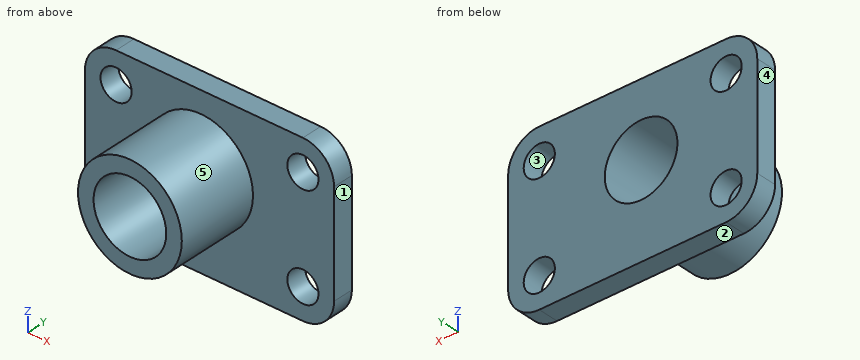
from build123d import *

# Parameters (mm, degrees)
F0_R     = 25
F0_R_2   = 17.5
F1_DEPTH = 50
F2_DEPTH = 112
F0_R_3   = 7.5
F3_DEPTH = 10


# Not quite as in the source:
# - an extrude ends at something that could not be found from the text; its depth is read off the source's solid


with BuildPart() as f1:
    # F0 (on Front) → F1 (new body)
    with BuildSketch(Plane.XZ):
        Circle(F0_R)
        Circle(F0_R_2, mode=Mode.SUBTRACT)
    extrude(amount=F1_DEPTH)

    # F0 (on Front) → F2 (cut, through all)
    with BuildSketch(Plane.XZ):
        Circle(F0_R_2)
    extrude(amount=-F2_DEPTH, mode=Mode.SUBTRACT)

    # F0 (on Front) → F3 (join)
    with BuildSketch(Plane.XZ):
        with BuildLine():
            Line((49.0495060384, 35.4441977432), (-40.9504939616, 35.4441977432))
            ThreePointArc((-40.9504939616, 35.4441977432), (-51.5570956794, 31.050799461), (-55.9504939616, 20.4441977432))
            Line((-55.9504939616, 20.4441977432), (-55.9504939616, -29.5558022568))
            ThreePointArc((-55.9504939616, -29.5558022568), (-51.5570956794, -40.1624039746), (-40.9504939616, -44.5558022568))
            Line((-40.9504939616, -44.5558022568), (49.0495060384, -44.5558022568))
            ThreePointArc((49.0495060384, -44.5558022568), (59.6561077562, -40.1624039746), (64.0495060384, -29.5558022568))
            Line((64.0495060384, -29.5558022568), (64.0495060384, 20.4441977432))
            ThreePointArc((64.0495060384, 20.4441977432), (59.6561077562, 31.050799461), (49.0495060384, 35.4441977432))
        make_face()
        with Locations((-40.9504939616, -29.5558022568)):
            Circle(F0_R_3, mode=Mode.SUBTRACT)
        with Locations((49.0495060384, -29.5558022568)):
            Circle(F0_R_3, mode=Mode.SUBTRACT)
        Circle(F0_R, mode=Mode.SUBTRACT)
        with Locations((-40.9504939616, 20.4441977432)):
            Circle(F0_R_3, mode=Mode.SUBTRACT)
        with Locations((49.0495060384, 20.4441977432)):
            Circle(F0_R_3, mode=Mode.SUBTRACT)
    extrude(amount=F3_DEPTH)


solid = f1.part
Verification items for the finished model (mm, model axes). Face numbers are marked on the shaded views. A direction names the side the tool comes from. Round coordinates to 2 decimals unless told otherwise and drop trailing zeros. Loops run counter-clockwise (first coordinate to the right, second up) from the corner with the lowest first, then second, coordinate; pieces in that order, holes last. Notation, with made-up numbers: (1, 3) - (45, 3) arc R14 cw to (45, 7) - close; hole circle Ø1 at (39.25, 63). An arc over 180 degrees is marked (long way). Use a Markdown table: item, result. Add a question column.
1. Section check C-C, the plane y = -4.5. Record the boundary of the cut face in (x, z).
2. Gauge pin test, flat ends, axial feed: pin 1 (2 mm diameter, centred on x = 18.5, y = -32, fed in from +Z); pin 2 (13.5 mm diameter, centred on x = -40.95, z = -29.56, fed in from -Y); pin 3 (10 mm diameter, centred on x = -9, y = -34, fed in from -Z); pin 4 (12 mm diameter, centred on x = 3.5, y = -36, fed in from +Z). Record the tip position at first contact, or that the pin passes through.
3. Access from +Z, -Z, +X, -X, +Y, -Y to the whole of each face (thin tool, end or side, straight path). Record for the marked faces 4 and 5.
4. Section check A-A, the plane z = 0. Record the boundary of the cut face in (x, y), plus the area to 3 significant figures.
5. Release check for a two-part mould opening along Z. For the marked faces 1, 2 and 3 record: released by +Z, released by -Z, zero draft, split by the parting line, or undercut.
6. Section check D-D, the plane y = -19. Record the boundary of the cut face in (x, z).
7. Section check B-B, the plane x = 0. Record the boundary of the cut face in (y, z), plus the area to 3 significant figures.
8. Thickness scan on probe 1 along Z at (x, y) = (-41.5, -3.5); probe 2 along Z at (x, y) = (0, -11.5); probe 3 along Z at (x, y) = (44.5, -7.5). Record the ranges inside material, lowest first. Write a range as [from, to].
Checks:
| question | item | result |
|---|---|---|
| 1 | outline | (-55.95, -29.56) arc R15 ccw to (-40.95, -44.56) - (49.05, -44.56) arc R15 ccw to (64.05, -29.56) - (64.05, 20.44) arc R15 ccw to (49.05, 35.44) - (-40.95, 35.44) arc R15 ccw to (-55.95, 20.44) - close; hole circle Ø15 at (-40.95, -29.56); hole circle Ø15 at (-40.95, 20.44); hole circle Ø35 at (0, 0); hole circle Ø15 at (49.05, -29.56); hole circle Ø15 at (49.05, 20.44) |
| 2 | pin 1 | stops at z = 17.85 |
| 2 | pin 2 | passes through |
| 2 | pin 3 | stops at z = -24.68 |
| 2 | pin 4 | stops at z = 25 |
| 3 | face 4 | +Z, -Z, -X, +Y, -Y |
| 3 | face 5 | -Y |
| 4 | outline | (-55.95, -10) - (-25, -10) - (-25, -50) - (-17.5, -50) - (-17.5, 0) - (-55.95, 0) - close; (17.5, -50) - (25, -50) - (25, -10) - (64.05, -10) - (64.05, 0) - (17.5, 0) - close |
| 4 | area | 1,450 mm^2 |
| 5 | face 1 | zero draft |
| 5 | face 2 | released by -Z |
| 5 | face 3 | undercut |
| 6 | outline | circle Ø50 at (0, 0); hole circle Ø35 at (0, 0) |
| 7 | outline | (-50, -25) - (-10, -25) - (-10, -44.56) - (0, -44.56) - (0, -17.5) - (-50, -17.5) - close; (-50, 17.5) - (0, 17.5) - (0, 35.44) - (-10, 35.44) - (-10, 25) - (-50, 25) - close |
| 7 | area | 1,050 mm^2 |
| 8 | probe 1 | z = [-44.55, -37.04], [-22.08, 12.96], [27.92, 35.43] |
| 8 | probe 2 | z = [-25, -17.5], [17.5, 25] |
| 8 | probe 3 | z = [-44.56, -35.52], [-23.59, 14.48], [26.41, 35.44] |
